Source: three-view drawing plus pictorial views. Frame: mm from the lowest corner of the part. A direction names the side the tool comes from. Give positions to 0.01 mm unless a question says otherwise; leave off trailing zeros. Order: outer loops, then holes, each group sorted by start corner. A loop starts at its lowest first (then second) coordinate and runs counter-clockwise, first axis right, second up.
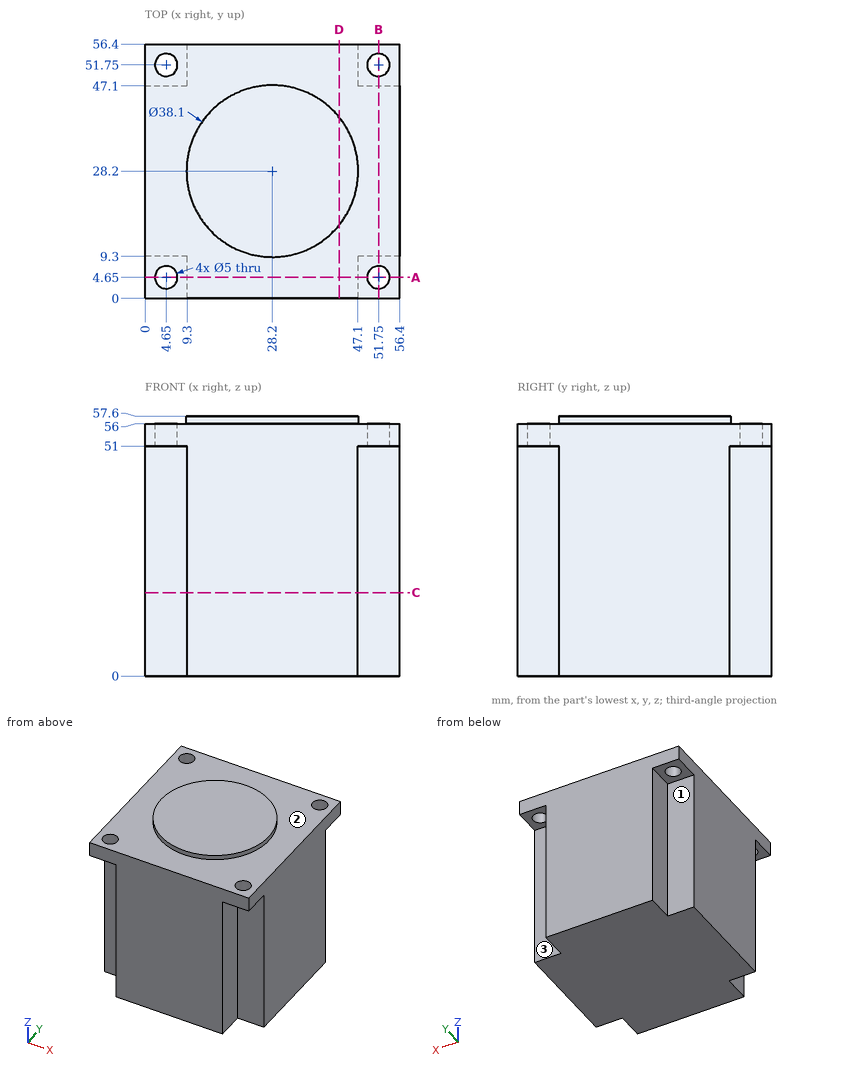
1) Ray query, L1, parallel to Y at x = 4.65, z = 55.05; L2, parallel to X at y = 53, z = 53.5; L3, parallel to Z at x = 10, y = 40. Return the intervals inside material, ascending.
Checks:
L1: y = 0 to 2.15, 7.15 to 49.25, 54.25 to 56.4
L2: x = 0 to 2.48, 6.82 to 49.58, 53.92 to 56.4
L3: z = 0 to 56
2) Section query C-C on z = 18.5. Output: boundary loops of the cut face in (x, y), and give its area (4 significant figures).
Checks:
outline: (0, 9.3) - (9.3, 9.3) - (9.3, 0) - (47.1, 0) - (47.1, 9.3) - (56.4, 9.3) - (56.4, 47.1) - (47.1, 47.1) - (47.1, 56.4) - (9.3, 56.4) - (9.3, 47.1) - (0, 47.1) - close
area: 2,835 mm2
3) Section query D-D on x = 43. Output: boundary loops of the cut face in (y, z), and give its area (3 significant figures).
Checks:
outline: (0, 0) - (56.4, 0) - (56.4, 56) - (40.19, 56) - (40.19, 57.6) - (16.21, 57.6) - (16.21, 56) - (0, 56) - close
area: 3,200 mm2
4) Reachability of the marked faces 1, 2 and 3 from +Z, -Z, +X, -X, +Y, -Y: full face, straight path, thin tool, end or side. Return the list, or none.
Checks:
face 1: -Z, -X, +Y
face 2: +Z
face 3: -Z, +X, +Y
5) Section query A-A on y = 4.65. Output: boundary loops of the cut face in (x, z).
Checks:
outline: (0, 51) - (2.15, 51) - (2.15, 56) - (0, 56) - close; (7.15, 51) - (9.3, 51) - (9.3, 0) - (47.1, 0) - (47.1, 51) - (49.25, 51) - (49.25, 56) - (7.15, 56) - close; (54.25, 51) - (56.4, 51) - (56.4, 56) - (54.25, 56) - close
6) First-contact query: pin 1 Ø4.5 at (x, z) = (50.5, 22) entering from -Y; pin 2 Ø3 at (y, z) = (53.5, 14) entering from -X; pin 3 Ø8 at (x, y) = (4.65, 51.75) entering from -Z. Flat tips, straight axial feed; report the tip coordinate or a pass-through.
Checks:
pin 1: stops at y = 9.3
pin 2: stops at x = 9.3
pin 3: stops at z = 51
